Here's how the part is built. I have some questions about the finished solid (model axes, mm). Face numbers are marked on the shaded views. A direction names the side the tool comes from. Give positions to 0.01 mm unless a question says otherwise; leave off trailing zeros. Write each loop counter-clockwise with the first axis right and the second up, starting at its lowest first coordinate (ties: lowest second). Pieces come first, ordered by that corner, then holes. Notation, with made-up numbers: (21.5, 33.25) -> (59.5, 33.25) arc R19 ccw to (59.5, 68.25) -> close; hole circle Ø3 at (17.25, 82.25). An arc over 180 degrees is marked (long way). Return JSON: item names as keys, results as strings.
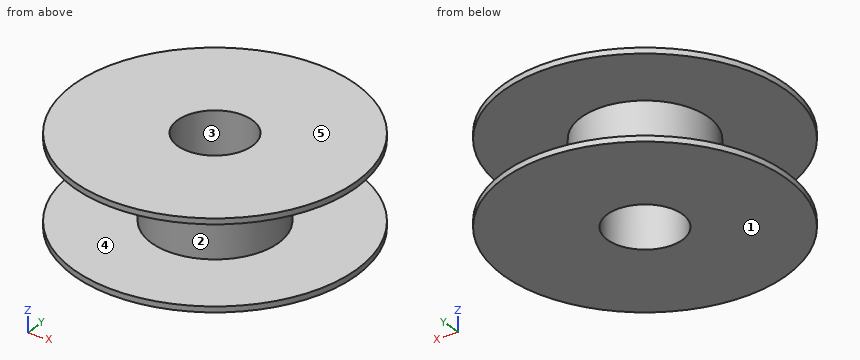
from build123d import *

# Parameters (mm, degrees)
SKETCH1_R           = 100
SKETCH1_R_2         = 26.5
BOSS_EXTRUDE1_DEPTH = 31.5
SKETCH2_R           = 100
SKETCH2_R_2         = 45
CUT_EXTRUDE1_DEPTH  = 27.5


with BuildPart() as part:
    # Sketch1 → Boss-Extrude1 (new, symmetric)
    with BuildSketch(Plane.XY):
        Circle(SKETCH1_R)
        Circle(SKETCH1_R_2, mode=Mode.SUBTRACT)
    extrude(amount=BOSS_EXTRUDE1_DEPTH, both=True)

    # Sketch2 → Cut-Extrude1 (cut, symmetric)
    with BuildSketch(Plane.XY):
        Circle(SKETCH2_R)
        Circle(SKETCH2_R_2, mode=Mode.SUBTRACT)
    extrude(amount=CUT_EXTRUDE1_DEPTH, both=True, mode=Mode.SUBTRACT)


solid = part.part
1. If I drill on line 1 (Y direction, x = 0, z = -14.5); line 2 (Z direction, x = -73, y = -62); line 3 (Y direction, x = 6.5, z = 29), over which ranges is the centre line in solid material (lowest first)? Write a range as [from, to].
Taken from the geometry:
{"line 1": "y = [-45, -26.5], [26.5, 45]", "line 2": "z = [-31.5, -27.5], [27.5, 31.5]", "line 3": "y = [-99.79, -25.69], [25.69, 99.79]"}
2. If we mould it in two halves opening along X, with no side actions, what happens to the marked faces 1, 2 and 3? For each: released by +X, released by -X, zero draft, split by the parting line, or undercut.
Taken from the geometry:
{"face 1": "zero draft", "face 2": "split by the parting line", "face 3": "undercut"}
3. For pin 1 Ø12 at (x, z) = (15.5, 20.5) entering from +Y; pin 2 Ø8 at (x, z) = (-35.5, -13) entering from -Y; pin 3 Ø5 at (x, z) = (-15, -7.5) entering from +Y, each with a flat end and sliding along its axis, tell me the tip position at first contact or that it passes through.
Taken from the geometry:
{"pin 1": "stops at y = 43.99", "pin 2": "stops at y = -32.14", "pin 3": "stops at y = 43.23"}
4. Suppose I cut it at D-D, the plane x = -51.5. List the corners of the cut face in (y, z) for me, and give its area (3 significant figures).
Taken from the geometry:
{"outline": "(-85.72, -31.5) -> (85.72, -31.5) -> (85.72, -27.5) -> (-85.72, -27.5) -> close; (-85.72, 27.5) -> (85.72, 27.5) -> (85.72, 31.5) -> (-85.72, 31.5) -> close", "area": "1,370 mm²"}
5. Which directions (+Z, -Z, +X, -X, +Y, -Y) give clear straight access to the entire face, cutting with the end or side of a thin tool? Please do the marked faces 4 and 5.
Taken from the geometry:
{"face 4": "none", "face 5": "+Z, +X, -X, +Y, -Y"}
6. Suppose I cut it at A-A, the plane y = 0. List the corners of the cut face in (x, z) for me, and give its area (3 significant figures).
Taken from the geometry:
{"outline": "(-100, -31.5) -> (-26.5, -31.5) -> (-26.5, 31.5) -> (-100, 31.5) -> (-100, 27.5) -> (-45, 27.5) -> (-45, -27.5) -> (-100, -27.5) -> close; (26.5, -31.5) -> (100, -31.5) -> (100, -27.5) -> (45, -27.5) -> (45, 27.5) -> (100, 27.5) -> (100, 31.5) -> (26.5, 31.5) -> close", "area": "3,210 mm²"}
7. Suppose I cut it at C-C, the plane z = -11. List the corners of the cut face in (x, y) for me, and give its area (3 significant figures).
Taken from the geometry:
{"outline": "circle Ø90 at (0, 0); hole circle Ø53 at (0, 0)", "area": "4,160 mm²"}
